from build123d import *

# Parameters (mm, degrees)
SKIZZE1_R                       = 4.57
SKIZZE1_R_2                     = 2
AUFSATZ_LINEAR_AUSTRAGEN1_DEPTH = 6.7
SCHNITT_LINEAR_AUSTRAGEN1_DEPTH = 7.7
VERRUNDUNG1_R                   = 0.5
KREISMUSTER1_COUNT              = 10
VERRUNDUNG1_OF_KREISMUSTER1_R   = 0.5
FASE2_SIZE                      = 0.2


with BuildPart() as part:
    # Skizze1 → Aufsatz-Linear austragen1 (new body)
    with BuildSketch(Plane(origin=(0, 0, 0), x_dir=(1, 0, 0), z_dir=(0, 1, 0))):
        Circle(SKIZZE1_R)
        Circle(SKIZZE1_R_2, mode=Mode.SUBTRACT)
    extrude(amount=AUFSATZ_LINEAR_AUSTRAGEN1_DEPTH)

    # Skizze12 → Schnitt-Linear austragen1 (cut, through all)
    with BuildSketch(Plane(origin=(0, 6.7, 0), x_dir=(1, 0, 0), z_dir=(0, 1, 0))):
        with BuildLine():
            Line((-1.2, 4.409637173), (-0.808470756, 3.57))
            Line((-0.808470756, 3.57), (0.808470756, 3.57))
            Line((0.808470756, 3.57), (1.2, 4.409637173))
            ThreePointArc((1.2, 4.409637173), (0, 4.57), (-1.2, 4.409637173))
        make_face()
    schnitt_linear_austragen1 = extrude(amount=-SCHNITT_LINEAR_AUSTRAGEN1_DEPTH, mode=Mode.SUBTRACT)

    # Verrundung1
    verrundung1_edges = [part.edges().sort_by_distance(p)[0] for p in [
        (0.808470756, 3.35, -3.57),
        (-0.808470756, 3.35, -3.57),
    ]]
    fillet(verrundung1_edges, radius=VERRUNDUNG1_R)

    # Kreismuster1: Schnitt-Linear austragen1 ×10 about axis
    kreismuster1_axis = Axis((0, 0, 0), (0, 1, 0))
    for i in range(1, KREISMUSTER1_COUNT):
        add(schnitt_linear_austragen1.rotate(kreismuster1_axis, i * 360 / KREISMUSTER1_COUNT), mode=Mode.SUBTRACT)

    # Verrundung1 of Kreismuster1
    verrundung1_of_kreismuster1_edges = [part.edges().sort_by_distance(p)[0] for p in [
        (-1.44432677, 3.35, -3.363397857),
        (-2.752459932, 3.35, -2.412983483),
        (-3.14544056, 3.35, -1.872092051),
        (-3.645102966, 3.35, -0.334289289),
        (-3.645102966, 3.35, 0.334289289),
        (-3.14544056, 3.35, 1.872092051),
        (-2.752459932, 3.35, 2.412983483),
        (-1.44432677, 3.35, 3.363397857),
        (-0.808470756, 3.35, 3.57),
        (0.808470756, 3.35, 3.57),
        (1.44432677, 3.35, 3.363397857),
        (2.752459932, 3.35, 2.412983483),
        (3.14544056, 3.35, 1.872092051),
        (3.645102966, 3.35, 0.334289289),
        (3.645102966, 3.35, -0.334289289),
        (3.14544056, 3.35, -1.872092051),
        (2.752459932, 3.35, -2.412983483),
        (1.44432677, 3.35, -3.363397857),
    ]]
    fillet(verrundung1_of_kreismuster1_edges, radius=VERRUNDUNG1_OF_KREISMUSTER1_R)

    # Fase2
    fase2_edges = [part.edges().sort_by_distance(p)[0] for p in [
        (-2, 0, 0),
        (-2, 6.7, 0),
    ]]
    chamfer(fase2_edges, length=FASE2_SIZE)


solid = part.part
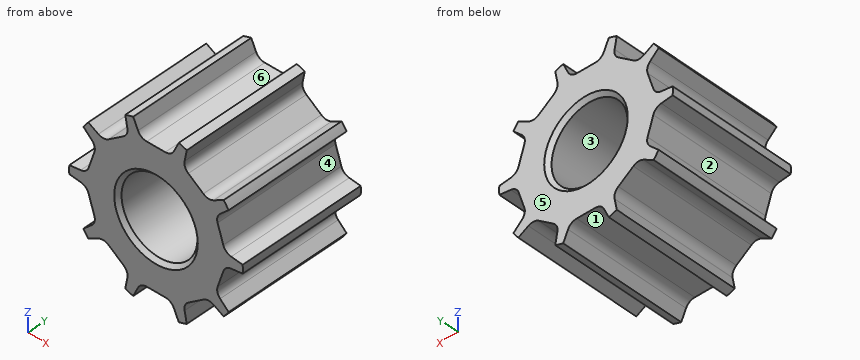
The model under review builds one solid part; all positions refer to its coordinate system, in mm. Face numbers are marked on the shaded views. A direction names the side the tool comes from. Coordinates: 2 decimals unless noted, no trailing zeros. Loops run counter-clockwise (first coordinate to the right, second up) from the corner with the lowest first, then second, coordinate; pieces in that order, holes last.
(1) Draft analysis for pull direction Z (two halves, no side actions). For the marked faces 4, 5 and 6, state which applies: +Z half, -Z half, draft (parallel to the pull), parting line (faces both ways), or undercut.
Determined:
face 4: undercut
face 5: draft
face 6: +Z half
(2) Insertion check: P1, Ø0.5, axis at x = 0, y = 3.5, coming from the +Z side; P2, Ø3, axis at y = 5, z = 3, coming from the -X side; P3, Ø4, axis at y = 4, z = 3, coming from the +X side; P4, Ø3.5, axis at x = 0, z = 0, coming from the +Y side. Each pin has a flat end and moves straight along its axis. Give the tip position at first contact, or say it passes through.
Determined:
P1: stops at z = 3.57
P2: stops at x = -3.82
P3: stops at x = 3.82
P4: passes through
(3) Tool access review of the marked faces 1, 2 and 3: name each direction out of +Z, -Z, +X, -X, +Y, -Y from which nothing blocks a thin tool from reaching the whole face with its end or side.
Determined:
face 1: -Z, +Y, -Y
face 2: -X, +Y, -Y
face 3: +Y, -Y
(4) Consider section B-B, the plane z = 0. Give the boundary of the cut face in (x, y), plus the area to 3 significant figures.
Determined:
outline: (-4.57, 0) - (-2.2, 0) - (-2, 0.2) - (-2, 6.5) - (-2.2, 6.7) - (-4.57, 6.7) - close; (2, 0.2) - (2.2, 0) - (4.57, 0) - (4.57, 6.7) - (2.2, 6.7) - (2, 6.5) - close
area: 34.4 mm2
(5) Consider section A-A, the plane x = 0. Give the boundary of the cut face in (y, z).
Determined:
outline: (0, -3.57) - (6.7, -3.57) - (6.7, -2.2) - (6.5, -2) - (0.2, -2) - (0, -2.2) - close; (0, 2.2) - (0.2, 2) - (6.5, 2) - (6.7, 2.2) - (6.7, 3.57) - (0, 3.57) - close
(6) Consider section C-C, the plane z = 3. Give the boundary of the cut face in (x, y), plus the area to 3 significant figures.
Determined:
outline: (-1.94, 0) - (1.94, 0) - (1.94, 6.7) - (-1.94, 6.7) - close
area: 26.1 mm2
(7) Wall thickness on L1, parallel to Z at x = 0, y = 5; L2, parallel to X at y = 3.5, z = 0; L3, parallel to X at y = 5.75, z = -2.75: over which ranges is each line inside the solid? List them lowest first.
Determined:
L1: z = -3.57 to -2, 2 to 3.57
L2: x = -4.57 to -2, 2 to 4.57
L3: x = -3.65 to -3.36, -2.29 to 2.29, 3.36 to 3.65
